```python
from build123d import *

# Parameters (mm, degrees)
SKETCH1_R           = 3
BOSS_EXTRUDE1_DEPTH = 10
CUT_EXTRUDE1_START  = -2
CUT_EXTRUDE1_DEPTH  = 2


with BuildPart() as part:
    # Sketch1 → Boss-Extrude1 (new body)
    with BuildSketch(Plane.XY):
        with BuildLine():
            Line((-8.75, 15.155444566), (-4, 19.905444566))
            Line((-4, 19.905444566), (-4, 22.905444566))
            ThreePointArc((-4, 22.905444566), (0, 26.905444566), (4, 22.905444566))
            Line((4, 22.905444566), (4, 19.905444566))
            Line((4, 19.905444566), (8.75, 15.155444566))
            ThreePointArc((8.75, 15.155444566), (0, 17.5), (-8.75, 15.155444566))
        make_face()
        with Locations((0, 22.905444566)):
            Circle(SKETCH1_R, mode=Mode.SUBTRACT)
    extrude(amount=BOSS_EXTRUDE1_DEPTH)

    # Sketch3 → Cut-Extrude1 (cut)
    with BuildSketch(Plane.XY.offset(10).offset(CUT_EXTRUDE1_START)):
        with BuildLine():
            ThreePointArc((0.75, 20.000707057), (0.378012877, 19.929355477), (0, 19.905444566))
            Line((0, 19.905444566), (0, 18.799598559))
            Line((0, 18.799598559), (0.75, 18.799598559))
            Line((0.75, 18.799598559), (0.75, 20.000707057))
        make_face()
        with BuildLine():
            Line((0, 18.799598559), (0, 19.905444566))
            ThreePointArc((0, 19.905444566), (-0.378012877, 19.929355477), (-0.75, 20.000707057))
            Line((-0.75, 20.000707057), (-0.75, 18.799598559))
            Line((-0.75, 18.799598559), (0, 18.799598559))
        make_face()
        with BuildLine():
            Line((0.75, 18.799598559), (0, 18.799598559))
            Line((0, 18.799598559), (0, 17.5))
            ThreePointArc((0, 17.5), (0.375086166, 17.495979834), (0.75, 17.483921185))
            Line((0.75, 17.483921185), (0.75, 18.799598559))
        make_face()
        with BuildLine():
            Line((0, 17.5), (0, 18.799598559))
            Line((0, 18.799598559), (-0.75, 18.799598559))
            Line((-0.75, 18.799598559), (-0.75, 17.483921185))
            ThreePointArc((-0.75, 17.483921185), (-0.375086166, 17.495979834), (0, 17.5))
        make_face()
    extrude(amount=CUT_EXTRUDE1_DEPTH, mode=Mode.SUBTRACT)


solid = part.part
```
Can you work these out from the model? Positions are in its coordinate system, mm. A direction names the side the tool comes from. Round coordinates to 2 decimals unless told otherwise and drop trailing zeros. Loops run counter-clockwise (first coordinate to the right, second up) from the corner with the lowest first, then second, coordinate; pieces in that order, holes last. Notation, with made-up numbers: M -24,-7.75 L -7,-7.75 A19 ccw -7,2.25 Z; hole C -12,8.25 d2. An arc over 180 degrees is marked long. Answer as a JSON object with one key per item and string values. Group by question number.
Q1. Imagine slicing it at A-A, the plane x = 0. Please give me the cut outline in (y, z), then the cut area to 3 significant figures.
Q2. We'd pull the mould along X, two halves only. Please class faces 1 (the cylindrical face through (1.613, 25.435, 4.93)), 2 (the flat face through (-6.408, 17.497, 4.93)), 3 (the flat face through (1.3, 19.8, 10)), 4 (the flat face through (0, 19, 8)): +X half, -X half, draft (parallel to the pull), parting line (faces both ways), or undercut.
Q3. On a 3-axis mill with a long thin cutter (end or side, diameter ignored), from which of +Z, -Z, +X, -X, +Y, -Y can I reach the whole of each face in a straight line? I mean faces 5 (the flat face through (-4, 21, 5)), 6 (the flat face through (4, 21, 5)), 7 (the flat face through (-0.75, 19, 9)). Say none if no direction works.
Q4. Imagine slicing it at C-C, the plane y = 21.5. Please give me the cut outline in (x, z).
Q5. Imagine slicing it at B-B, the plane z = 3.5. Please give me the cut outline in (x, y), then the cut area to 3 significant figures.
Q6. Imagine slicing it at D-D, the plane z = 8.25. Please give me the cut outline in (x, y), then the cut area to 3 significant figures.
Q7. Please list where these lines run through material, in increasing order: L1, parallel to Y at x = 0, z = 5; L2, parallel to X at y = 23, z = 7.5; L3, parallel to X at y = 23.5, z = 1.75.
Q8. Will these pins go through, and if not, where does the flat tip stop? pin 1 (1.5 mm diameter, centred on x = -5.5, z = 7.5, fed in from +Y); pin 2 (3 mm diameter, centred on y = 20.5, z = 8, fed in from -X); pin 3 (1.5 mm diameter, centred on x = -1, z = 2.5, fed in from -Y).
Findings:
{
 "1": {"outline": "M 17.5,0 L 19.91,0 L 19.91,8 L 17.5,8 Z; M 25.91,0 L 26.91,0 L 26.91,10 L 25.91,10 Z", "area": "29.2 mm2"},
 "2": {"face 1": "undercut", "face 2": "-X half", "face 3": "draft", "face 4": "undercut"},
 "3": {"face 5": "+Z, -Z, -X, +Y", "face 6": "+Z, -Z, +X, +Y", "face 7": "+Z, -Y"},
 "4": {"outline": "M -4,0 L -2.65,0 L -2.65,10 L -4,10 Z; M 2.65,0 L 4,0 L 4,10 L 2.65,10 Z"},
 "5": {"outline": "M -8.75,15.16 A17.5 cw 8.75,15.16 L 4,19.91 L 4,22.91 A4 ccw -4,22.91 L -4,19.91 Z; hole C 0,22.91 d6", "area": "53.7 mm2"},
 "6": {"outline": "M -8.75,15.16 A17.5 cw -0.75,17.48 L -0.75,20 A3 cw long 0.75,20 L 0.75,17.48 A17.5 cw 8.75,15.16 L 4,19.91 L 4,22.91 A4 ccw -4,22.91 L -4,19.91 Z", "area": "50.0 mm2"},
 "7": {"L1": "y = 17.5 to 19.91, 25.91 to 26.91", "L2": "x = -4 to -3, 3 to 4", "L3": "x = -3.96 to -2.94, 2.94 to 3.96"},
 "8": {"pin 1": "stops at y = 19.16", "pin 2": "stops at x = -4.91", "pin 3": "stops at y = 17.41"}
}
